```python
from build123d import *

# Parameters (mm, degrees)
SKETCH5_W               = 38.1
SKETCH5_H               = 298.45
BOSS_EXTRUDE2_DEPTH     = 19.05
F_3_8_CLEARANCE_HOLE2_D = 10.31748
F_3_8_CLEARANCE_HOLE4_D = 13.97
BODY_MOVE_COPY4_ANGLE   = 90
F_3_8_CLEARANCE_HOLE3_D = 10.31748
CUT_EXTRUDE1_DEPTH      = 218.574389578
CUT_EXTRUDE1_DEPTH_BACK = 218.574389578
CUT_EXTRUDE2_DEPTH      = 218.574389578
CUT_EXTRUDE2_DEPTH_BACK = 218.574389578
SKETCH12_W              = 25.4
SKETCH12_H              = 37.531383446
SKETCH12_H_2            = 37.531383447
CUT_EXTRUDE3_DEPTH      = 218.574389578
CUT_EXTRUDE3_DEPTH_BACK = 218.574389578
CUT_EXTRUDE5_DEPTH      = 211.093240097
CUT_EXTRUDE5_DEPTH_BACK = 211.093240097
FILLET1_R               = 3.175
FILLET2_R               = 6.35
FILLET3_R               = 6.35


with BuildPart() as part:
    # Sketch5 → Boss-Extrude2 (new, symmetric)
    with BuildSketch(Plane.XY):
        with Locations((0, 66.675)):
            Rectangle(SKETCH5_W, SKETCH5_H)
    extrude(amount=BOSS_EXTRUDE2_DEPTH, both=True)

    # 3/8 Clearance Hole2 (through all)
    with Locations(Plane(origin=(19.05, 0, 0), x_dir=(0, 0, -1), z_dir=(1, 0, 0))):
        with Locations((0, -57.15)):
            Hole(F_3_8_CLEARANCE_HOLE2_D / 2)

    # 3/8 Clearance Hole4 (through all)
    with Locations(Plane(origin=(19.05, 0, 0), x_dir=(0, 0, -1), z_dir=(1, 0, 0))):
        with Locations((0, 0)):
            Hole(F_3_8_CLEARANCE_HOLE4_D / 2)


with BuildPart() as body_2:
    # uxcell-FR6ZZ: read off the stored shape, not the designer's step
    # uxcell-FR6ZZ outline → uxcell-FR6ZZ (revolve)
    with BuildSketch(Plane(origin=(46.870492888, 0, -67.456601715), x_dir=(1, 0, 0), z_dir=(0, 0, 1))):
        Polygon((12.303125, 146.229545606), (4.7625, 146.229545606), (4.7625, 138.704795606), (11.1125, 138.704795606), (11.1125, 143.864170606), (11.509375, 144.261045606), (12.303125, 144.261045606), align=None)
    revolve(axis=Axis((46.870492888, 0, -67.456601715), (0, 1, 0)))


with BuildPart() as body_2_1:
    # Body-Move/Copy4: read off the stored shape, not the designer's step
    # Body-Move/Copy4: moved
    add(body_2.part.moved(Location((-46.8704929, -127.1795456, 67.4566017))).rotate(Axis((0, 0, 0), (0, 0, -1)), BODY_MOVE_COPY4_ANGLE))


with BuildPart() as body_3:
    # Mirror1: mirrored copy
    add(body_2_1.part.mirror(Plane(origin=(0, 0, 0), x_dir=(0, 0, 1), z_dir=(1, 0, 0))))


with BuildPart() as part_1:
    add(part.part)

    # Combine2: cut body 3, body 2
    add(body_3.part, mode=Mode.SUBTRACT)
    add(body_2_1.part, mode=Mode.SUBTRACT)

    # 3/8 Clearance Hole3 (through all)
    with Locations(Plane(origin=(19.05, 0, 0), x_dir=(0, 0, -1), z_dir=(1, 0, 0))):
        with Locations((-9.525, 196.85), (9.525, 196.85)):
            Hole(F_3_8_CLEARANCE_HOLE3_D / 2)

    # Sketch11 → Cut-Extrude1 (cut, two sides: drawn at the far end of the back side and taken through both)
    with BuildSketch(Plane.XY.offset(-CUT_EXTRUDE1_DEPTH_BACK)):
        Polygon((-6.35, -691.607801887), (-6.35, -82.55), (-6.35, -31.75), (19.05, -25.4), (609.922858655, 122.318214664), (1581.067185153, -612.994182394), (964.794326498, -1426.920198945), align=None)
    extrude(amount=CUT_EXTRUDE1_DEPTH + CUT_EXTRUDE1_DEPTH_BACK, mode=Mode.SUBTRACT)

    # Sketch12 → Cut-Extrude2 (cut, two sides: drawn at the far end of the back side and taken through both)
    with BuildSketch(Plane(origin=(0, 0, 0), x_dir=(0, 0, -1), z_dir=(1, 0, 0)).offset(-CUT_EXTRUDE2_DEPTH_BACK)):
        with Locations((0, 163.400568277)):
            Rectangle(SKETCH12_W, SKETCH12_H)
        with Locations((0, 121.106684831)):
            Rectangle(SKETCH12_W, SKETCH12_H_2)
        with Locations((0, 78.812801384)):
            Rectangle(SKETCH12_W, SKETCH12_H)
        with BuildLine():
            Line((12.7, 17.753226214), (12.7, 55.284609661))
            Line((12.7, 55.284609661), (-12.7, 55.284609661))
            Line((-12.7, 55.284609661), (-12.7, 17.753226214))
            ThreePointArc((-12.7, 17.753226214), (0, 21.828125), (12.7, 17.753226214))
        make_face()
    extrude(amount=CUT_EXTRUDE2_DEPTH + CUT_EXTRUDE2_DEPTH_BACK, mode=Mode.SUBTRACT)

    # Sketch16 → Cut-Extrude3 (cut, two sides: drawn at the far end of the back side and taken through both)
    with BuildSketch(Plane(origin=(0, 0, 0), x_dir=(0, 0, -1), z_dir=(1, 0, 0)).offset(-CUT_EXTRUDE3_DEPTH_BACK)):
        Polygon((-615.836179143, 208.35874), (-19.05, 208.35874), (19.05, 208.35874), (615.836179143, 208.35874), (615.836179143, 1401.931098287), (-615.836179143, 1401.931098287), align=None)
    extrude(amount=CUT_EXTRUDE3_DEPTH + CUT_EXTRUDE3_DEPTH_BACK, mode=Mode.SUBTRACT)

    # Sketch18 → Cut-Extrude5 (cut, two sides: drawn at the far end of the back side and taken through both)
    with BuildSketch(Plane(origin=(0, 0, 0), x_dir=(0, 0, -1), z_dir=(1, 0, 0)).offset(-CUT_EXTRUDE5_DEPTH_BACK)):
        Polygon((-66.072467933, 439.146371732), (-19.05, -8.242525716), (-12.7, -68.65874), (12.7, -68.65874), (19.05, -8.242525716), (66.072467933, 439.146371732), (66.072467933, -460.560109405), (-66.072467933, -460.560109405), align=None)
    extrude(amount=CUT_EXTRUDE5_DEPTH + CUT_EXTRUDE5_DEPTH_BACK, mode=Mode.SUBTRACT)

    # Fillet1
    fillet1_edges = [part_1.edges().sort_by_distance(p)[0] for p in [
        (0, 60.047109661, -12.7),
        (0, 60.047109661, 12.7),
        (0, 55.284609661, 12.7),
        (0, 55.284609661, -12.7),
        (0, 17.753226214, -12.7),
        (0, 17.753226214, 12.7),
        (0, 182.16626, -12.7),
        (0, 144.634876554, -12.7),
        (0, 144.634876554, 12.7),
        (0, 182.16626, 12.7),
        (0, 139.872376554, 12.7),
        (0, 139.872376554, -12.7),
        (0, 102.340993107, -12.7),
        (0, 102.340993107, 12.7),
        (0, 97.578493107, 12.7),
        (0, 97.578493107, -12.7),
    ]]
    fillet(fillet1_edges, radius=FILLET1_R)

    # Fillet2
    fillet2_edges = [part_1.edges().sort_by_distance(p)[0] for p in [
        (0, 208.35874, -19.05),
        (0, 208.35874, 19.05),
        (0, -8.242525716, 19.05),
        (-12.7, -68.65874, 12.7),
        (-12.7, -68.65874, -12.7),
        (0, -8.242525716, -19.05),
    ]]
    fillet(fillet2_edges, radius=FILLET2_R)

    # Fillet3
    fillet3_edges = [part_1.edges().sort_by_distance(p)[0] for p in [
        (-6.35, -31.75, 0),
        (19.05, -25.4, 0),
    ]]
    fillet(fillet3_edges, radius=FILLET3_R)


solid = part_1.part
```
Source: CAD feature listing. Evaluate the final solid. Frame: model axes, mm. A direction names the side the tool comes from. Round coordinates to 2 decimals unless told otherwise and drop trailing zeros. Write each loop counter-clockwise with the first axis right and the second up, starting at its lowest first coordinate (ties: lowest second). Pieces come first, ordered by that corner, then holes. Notation, with made-up numbers: M 74,-5 L 123,-5 A25 cw 123,16 Z; hole C 39.25,61 d7. An arc over 180 degrees is marked long. Answer as a JSON object with one key per item and string values. Group by question number.
(1) Section query A-A on y = 160.5. Output: boundary loops of the cut face in (x, z).
(2) First-contact query: pin 1 (22 mm diameter, centred on y = 0, z = 0, fed in from -X); pin 2 (15 mm diameter, centred on x = 8.5, z = 0, fed in from -Y); pin 3 (19.5 mm diameter, centred on y = 0, z = 0, fed in from +X). Flat tips, straight axial feed; report the tip coordinate or a pass-through.
(3) Reachability of faces 4 (the flat face through (0, 37, -12.7)), 5 (the flat face through (-4.5, -30.11, 16.75)), 6 (the flat face through (17.082, 11, 4)) from +Z, -Z, +X, -X, +Y, -Y: full face, straight path, thin tool, end or side. Return the list, or none.
(4) Ray query, line 1 (Z direction, x = -15.7, y = 0); line 2 (Z direction, x = -3, y = 196); line 3 (Y direction, x = -4.5, z = 1). Return the intervals inside material, ascending. Write a range as [from, to].
(5) Section query B-B on y = 196.85. Output: boundary loops of the cut face in (x, z), then the cut area to 3 significant figures.
(6) Mould query, pull axis Y, two halves, no side actions, for faces 1 (the flat face through (-11.525, 7.3, -0.2)), 2 (the flat face through (-6.35, -49, 0)), 3 (the flat face through (-4.5, -29.35, -16.83)). Classes: +Y half, -Y half, draft (parallel to the pull), parting line (faces both ways), or undercut.
(7) Section query C-C on x = -14. State how many separate pieces and enclosed holes the cut face has, then the cut area to 3 significant figures.
Computed values:
{
 "1": {"outline": "M -19.05,-19.05 L 19.05,-19.05 L 19.05,-12.7 L -19.05,-12.7 Z; M -19.05,12.7 L 19.05,12.7 L 19.05,19.05 L -19.05,19.05 Z"},
 "2": {"pin 1": "x = -11.53", "pin 2": "y = -29.91", "pin 3": "x = 11.53"},
 "3": {"face 4": "+X, -X", "face 5": "+Z, +X, -X, -Y", "face 6": "+X"},
 "4": {"line 1": "[-19.05, -11.11], [11.11, 19.05]", "line 2": "[-19.05, -14.61], [-4.44, 4.44], [14.61, 19.05]", "line 3": "[-32.23, -6.91], [6.91, 21.81], [55.28, 60.05], [97.58, 102.34], [139.87, 144.63], [182.17, 208.36]"},
 "5": {"outline": "M -19.05,-19.05 L 19.05,-19.05 L 19.05,-14.68 L -19.05,-14.68 Z; M -19.05,-4.37 L 19.05,-4.37 L 19.05,4.37 L -19.05,4.37 Z; M -19.05,14.68 L 19.05,14.68 L 19.05,19.05 L -19.05,19.05 Z", "area": "665 mm^2"},
 "6": {"face 1": "undercut", "face 2": "draft", "face 3": "-Y half"},
 "7": {"separate pieces": "1", "enclosed holes": "8", "area": "5,800 mm^2"}
}
